The model under review builds one solid part; all positions refer to its coordinate system, in mm. A direction names the side the tool comes from. Give positions to 0.01 mm unless a question says otherwise; leave off trailing zeros. Loops run counter-clockwise (first coordinate to the right, second up) from the corner with the lowest first, then second, coordinate; pieces in that order, holes last. Notation, with made-up numbers: M 46,-23.75 L 64,-23.75 A31 cw 64,3.25 Z; hole C -22.5,-38 d10. An arc over 180 degrees is marked long. Write item = value, one per line. Start each with the question number.
1. We need section A-A on z = 2. Give the boundary of the cut face in (x, y), then the cut area to 3 significant figures.
2. We need section C-C on y = 1.25. Give the boundary of the cut face in (x, z).
3. For pin 1 (6 mm diameter, centred on x = -7, y = 1, fed in from +Z); pin 2 (0.7 mm diameter, centred on y = 11.5, z = 4.5, fed in from +X); pin 3 (2 mm diameter, centred on x = 9.5, z = 2.5, fed in from +Y); pin 4 (2.5 mm diameter, centred on x = 0, y = -11, fed in from -Z), all flat-tipped, find the tip position at first contact; note any pin that passes through.
4. For faces 1 (the face through (-11.4, 1.2, 4)), 2 (the face through (11, -3, 6)), 3 (the face through (-11, 12, 8)), list the 3-axis set-ups (+Z, -Z, +X, -X, +Y, -Y) from which the entire face can be reached by the end or side of a thin tool; tool diameter is ignored.
5. Wall thickness on line 1 along Y through (x, z) = (8, 1.8) (3 decimals); line 2 along Y through (x, z) = (-8, 4.25) (3 decimals); line 3 along Y through (x, z) = (0, 4.25): over which ranges is each line inside the solid? List them lowest first. Write a range as from..to.
6. We need section B-B on z = 7.25. Give the boundary of the cut face in (x, y).
7. We need section D-D on y = -11.5. Give the boundary of the cut face in (x, z) (1 decimal).
8. Draft analysis for pull direction Y (two halves, no side actions). For faces 4 (the face through (8.699, 12.096, 3.346)), 5 (the face through (-11.8, 0, 4)), 6 (the face through (0, 14.8, 3)), state which applies: pulls with the +Y half, pulls with the -Y half, needs draft (parallel to the pull), parting line crosses it, or undercut.
from build123d import *

# Parameters (mm, degrees)
SKETCH1_W                               = 23.6
SKETCH1_H                               = 29.6
BASIC_DEPTH                             = 8
SKETCH2_R                               = 3.5
F_7_0_HOLE_ROTATING_MAGNET_DEPTH        = 21.549452547
SKETCH4_R                               = 1.6
SKETCH4_R_2                             = 1.3
MOUNTING_HOLES_2_05_2_5_DEPTH           = 21.549452547
R4_BASIC_R                              = 4
PCB_LEVEL_DEPTH                         = 1.4
PCB_CLEARANCE_DEPTH                     = 4.2
R2_1_PCB_CLEARANCE_R                    = 2.1
R2_75_PCB_CLEARANCE_R                   = 2.75
CUT_OUT_1_DEPTH                         = 0.8
CUT_OUT_RESET_SWITCH_DEPTH              = 0.8
SKETCH13_R                              = 1.05
F_2_05_PCB_MOUNTING_HOLE_FOR_M2_5_DEPTH = 21.045947221


with BuildPart() as part:
    # Sketch1 → Basic (new body)
    with BuildSketch(Plane.XY):
        Rectangle(SKETCH1_W, SKETCH1_H)
    extrude(amount=BASIC_DEPTH)

    # Sketch2 → Ø7.0 Hole (Rotating Magnet) (cut, through all)
    with BuildSketch(Plane.XY.offset(8)):
        with Locations((0, 9)):
            Circle(SKETCH2_R)
    extrude(amount=-F_7_0_HOLE_ROTATING_MAGNET_DEPTH, mode=Mode.SUBTRACT)

    # Sketch4 → Mounting holes  Ø2.05 & Ø2.5 (cut, through all)
    with BuildSketch(Plane.XY.offset(8)):
        with Locations((8, -11)):
            Circle(SKETCH4_R)
        with Locations((-8, -11)):
            Circle(SKETCH4_R)
        with Locations((8, 11)):
            Circle(SKETCH4_R_2)
        with Locations((-8, 11)):
            Circle(SKETCH4_R_2)
    extrude(amount=-MOUNTING_HOLES_2_05_2_5_DEPTH, mode=Mode.SUBTRACT)

    # R4: Basic
    r4_basic_edges = [part.edges().sort_by_distance(p)[0] for p in [
        (11.8, -14.8, 4),
        (-11.8, -14.8, 4),
        (-11.8, 14.8, 4),
        (11.8, 14.8, 4),
    ]]
    fillet(r4_basic_edges, radius=R4_BASIC_R)

    # Sketch6 → PCB level (cut)
    with BuildSketch(Plane.XY.offset(8)):
        with BuildLine():
            Line((11, -10.8), (11, 10.8))
            ThreePointArc((11, 10.8), (10.0627417, 13.0627417), (7.8, 14))
            Line((7.8, 14), (-7.8, 14))
            ThreePointArc((-7.8, 14), (-10.0627417, 13.0627417), (-11, 10.8))
            Line((-11, 10.8), (-11, -10.8))
            ThreePointArc((-11, -10.8), (-10.0627417, -13.0627417), (-7.8, -14))
            Line((-7.8, -14), (7.8, -14))
            ThreePointArc((7.8, -14), (10.0627417, -13.0627417), (11, -10.8))
        make_face()
    extrude(amount=-PCB_LEVEL_DEPTH, mode=Mode.SUBTRACT)

    # Sketch9 → PCB Clearance (cut)
    with BuildSketch(Plane.XY.offset(8)):
        with BuildLine():
            Line((-11, 8.25), (-5.25, 8.25))
            Line((-5.25, 8.25), (-5.25, 14))
            Line((-5.25, 14), (5.25, 14))
            Line((5.25, 14), (5.25, 8.25))
            Line((5.25, 8.25), (11, 8.25))
            Line((11, 8.25), (11, -10.8))
            ThreePointArc((11, -10.8), (10.0627417, -13.0627417), (7.8, -14))
            Line((7.8, -14), (2.875, -14))
            Line((2.875, -14), (2.875, -8.25))
            Line((2.875, -8.25), (-2.875, -8.25))
            Line((-2.875, -8.25), (-2.875, -14))
            Line((-2.875, -14), (-7.8, -14))
            ThreePointArc((-7.8, -14), (-10.0627417, -13.0627417), (-11, -10.8))
            Line((-11, -10.8), (-11, 8.25))
        make_face()
    extrude(amount=-PCB_CLEARANCE_DEPTH, mode=Mode.SUBTRACT)

    # R2.1: PCB Clearance
    r2_1_pcb_clearance_edges = [part.edges().sort_by_distance(p)[0] for p in [
        (-11, 8.25, 5.2),
        (-5.25, 14, 5.2),
        (5.25, 14, 5.2),
        (11, 8.25, 5.2),
        (2.875, -14, 5.2),
        (-2.875, -14, 5.2),
    ]]
    fillet(r2_1_pcb_clearance_edges, radius=R2_1_PCB_CLEARANCE_R)

    # R2.75: PCB Clearance
    r2_75_pcb_clearance_edges = [part.edges().sort_by_distance(p)[0] for p in [
        (-5.25, 8.25, 5.2),
        (5.25, 8.25, 5.2),
        (2.875, -8.25, 5.2),
        (-2.875, -8.25, 5.2),
    ]]
    fillet(r2_75_pcb_clearance_edges, radius=R2_75_PCB_CLEARANCE_R)

    # Sketch11 → Cut-Out (1) (cut)
    with BuildSketch(Plane(origin=(0, 14.8, 0), x_dir=(1, 0, 0), z_dir=(0, 1, 0))):
        with BuildLine():
            Line((-1.5, -8), (-1.5, -5.5))
            ThreePointArc((-1.5, -5.5), (0, -4), (1.5, -5.5))
            Line((1.5, -5.5), (1.5, -8))
            Line((1.5, -8), (-1.5, -8))
        make_face()
    extrude(amount=-CUT_OUT_1_DEPTH, mode=Mode.SUBTRACT)

    # Sketch12 → Cut-Out Reset Switch (cut)
    with BuildSketch(Plane.ZY.offset(11.8)):
        with BuildLine():
            Line((8, -0.25), (5.5, -0.25))
            ThreePointArc((5.5, -0.25), (4, 1.25), (5.5, 2.75))
            Line((5.5, 2.75), (8, 2.75))
            Line((8, 2.75), (8, -0.25))
        make_face()
    extrude(amount=-CUT_OUT_RESET_SWITCH_DEPTH, mode=Mode.SUBTRACT)

    # Sketch13 → Ø2.05 PCB Mounting Hole for M2.5 (cut, through all)
    with BuildSketch(Plane.XY.offset(6.6)):
        with Locations((0, -11)):
            Circle(SKETCH13_R)
    extrude(amount=-F_2_05_PCB_MOUNTING_HOLE_FOR_M2_5_DEPTH, mode=Mode.SUBTRACT)


solid = part.part
Final values:
q1.outline = M -11.8,-10.8 A4 ccw -7.8,-14.8 L 7.8,-14.8 A4 ccw 11.8,-10.8 L 11.8,10.8 A4 ccw 7.8,14.8 L -7.8,14.8 A4 ccw -11.8,10.8 Z; hole C -8,-11 d3.2; hole C -8,11 d2.6; hole C 0,9 d7; hole C 0,-11 d2.1; hole C 8,-11 d3.2; hole C 8,11 d2.6
q1.area = 616 mm²
q2.outline = M -11.8,0 L 11.8,0 L 11.8,8 L 11,8 L 11,3.8 L -11,3.8 L -11,4 L -11.8,4 Z
q3.pin_1 = 3.8
q3.pin_2 = 11.78
q3.pin_3 = 14.74
q3.pin_4 = 0
q4.face_1 = +Z, -X
q4.face_2 = +Z
q4.face_3 = +Z, +X, -X, +Y, -Y
q5.line_1 = -14.795..-12.6, -9.4..9.7, 12.3..14.795
q5.line_2 = -14.795..-13.994, 8.25..9.7, 12.3..14.795
q5.line_3 = -14.8..-12.05, -9.95..-8.25
q6.outline = M -11.8,-10.8 A4 ccw -7.8,-14.8 L 7.8,-14.8 A4 ccw 11.8,-10.8 L 11.8,10.8 A4 ccw 7.8,14.8 L 1.5,14.8 L 1.5,14 L 7.8,14 A3.2 cw 11,10.8 L 11,-10.8 A3.2 cw 7.8,-14 L -7.8,-14 A3.2 cw -11,-10.8 L -11,-0.25 L -11.8,-0.25 Z; M -11.8,2.75 L -11,2.75 L -11,10.8 A3.2 cw -7.8,14 L -1.5,14 L -1.5,14.8 L -7.8,14.8 A4 ccw -11.8,10.8 Z
q7.outline = M -11.7,0 L -9.5,0 L -9.5,3.8 L -10.9,3.8 L -10.9,8 L -11.7,8 Z; M -6.5,0 L -0.9,0 L -0.9,6.6 L -2.9,6.6 L -2.9,3.8 L -6.5,3.8 Z; M 0.9,0 L 6.5,0 L 6.5,3.8 L 2.9,3.8 L 2.9,6.6 L 0.9,6.6 Z; M 9.5,0 L 11.7,0 L 11.7,8 L 10.9,8 L 10.9,3.8 L 9.5,3.8 Z
q8.face_4 = undercut
q8.face_5 = needs draft
q8.face_6 = pulls with the +Y half
